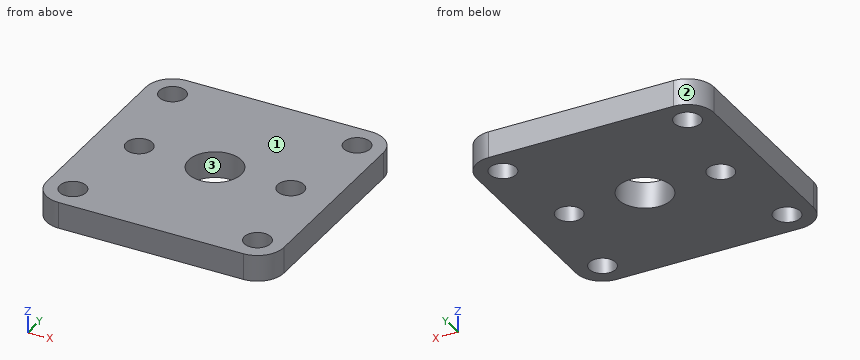
```python
from build123d import *

# Parameters (mm, degrees)
SKETCH_1_W      = 18
SKETCH_1_H      = 18
SKETCH_1_R      = 2
EXTRUDE_1_DEPTH = 2
MM_1_D          = 2
FILLET_1_R      = 2
MM_2_D          = 2


with BuildPart() as part:
    # 草图1 → 凸台-拉伸1 (new body)
    with BuildSketch(Plane.XY):
        Rectangle(SKETCH_1_W, SKETCH_1_H)
        Circle(SKETCH_1_R, mode=Mode.SUBTRACT)
    extrude(amount=EXTRUDE_1_DEPTH)

    # 大小mm 暗销孔1 (through all)
    with Locations(Plane(origin=(-7, 7, 2), x_dir=(1, 0, 0), z_dir=(0, 0, 1))):
        with Locations((0, 0), (14, 0), (14, -14), (0, -14)):
            Hole(MM_1_D / 2)

    # 圆角1
    fillet_1_edges = [part.edges().sort_by_distance(p)[0] for p in [
        (9, -9, 1),
        (-9, -9, 1),
        (-9, 9, 1),
        (9, 9, 1),
    ]]
    fillet(fillet_1_edges, radius=FILLET_1_R)

    # 大小mm 暗销孔2 (through all)
    with Locations(Plane(origin=(-5.75, 0, 2), x_dir=(1, 0, 0), z_dir=(0, 0, 1))):
        with Locations((0, 0), (11.5, 0)):
            Hole(MM_2_D / 2)


solid = part.part
```
Check sheet for the modelled part. Datum: model origin and axes. Units: mm. Face numbers are marked on the shaded views. Round coordinates to 2 decimals unless told otherwise and drop trailing zeros. Order: outer loops, then holes, each group sorted by start corner. A loop starts at its lowest first (then second) coordinate and runs counter-clockwise, first axis right, second up. Notation, with made-up numbers: (-4, 83) -> (27, 83) arc R14 cw to (27, 105) -> close; hole circle Ø6 at (-38, -13.5). An arc over 180 degrees is marked (long way). Use CSV: the item, a comma, the result in double quotes.
(1) Cross-section at D-D (x = -5.75). Record the boundary of the cut face in (y, z).
Worked out:
outline,"(-9, 0) -> (-1, 0) -> (-1, 2) -> (-9, 2) -> close; (1, 0) -> (9, 0) -> (9, 2) -> (1, 2) -> close"
(2) Cross-section at C-C (z = 0.4). Record the boundary of the cut face in (x, y), and give its area (3 significant figures).
Worked out:
outline,"(-9, -7) arc R2 ccw to (-7, -9) -> (7, -9) arc R2 ccw to (9, -7) -> (9, 7) arc R2 ccw to (7, 9) -> (-7, 9) arc R2 ccw to (-9, 7) -> close; hole circle Ø2 at (-7, -7); hole circle Ø2 at (-7, 7); hole circle Ø2 at (-5.75, 0); hole circle Ø4 at (0, 0); hole circle Ø2 at (5.75, 0); hole circle Ø2 at (7, -7); hole circle Ø2 at (7, 7)"
area,"289 mm²"
(3) Draft check along Y on the marked faces 1, 2 and 3. Enter one of: pulls with the +Y half, pulls with the -Y half, needs draft (parallel to the pull), parting line crosses it, or undercut.
Worked out:
face 1,"needs draft"
face 2,"pulls with the +Y half"
face 3,"undercut"
(4) Depth check by flat-ended pin: pin 1 (1.8 mm diameter, centred on x = -7, y = 7, fed in from -Z). Enter the tip coordinate at first touch or a pass-through.
Worked out:
pin 1,"through"
(5) Cross-section at B-B (y = 0). Record the boundary of the cut face in (x, z), and give its area (3 significant figures).
Worked out:
outline,"(-9, 0) -> (-6.75, 0) -> (-6.75, 2) -> (-9, 2) -> close; (-4.75, 0) -> (-2, 0) -> (-2, 2) -> (-4.75, 2) -> close; (2, 0) -> (4.75, 0) -> (4.75, 2) -> (2, 2) -> close; (6.75, 0) -> (9, 0) -> (9, 2) -> (6.75, 2) -> close"
area,"20.0 mm²"
(6) Material ranges on line 1 along Y through (x, z) = (-7, 0.8); line 2 along Y through (x, z) = (-5.75, 0.7); line 3 along X through (y, z) = (0.25, 1.7), recorded low to high. Write a range as from..to.
Worked out:
line 1,"-9..-8, -6..6, 8..9"
line 2,"-9..-1, 1..9"
line 3,"-9..-6.72, -4.78..-1.98, 1.98..4.78, 6.72..9"
(7) Cross-section at A-A (x = 0). Record the boundary of the cut face in (y, z), and give its area (3 significant figures).
Worked out:
outline,"(-9, 0) -> (-2, 0) -> (-2, 2) -> (-9, 2) -> close; (2, 0) -> (9, 0) -> (9, 2) -> (2, 2) -> close"
area,"28.0 mm²"
